Read the model definition and answer for the solid it produces. Units are mm, in the model's axes. Give positions to 0.01 mm unless a question says otherwise; leave off trailing zeros. Write each loop counter-clockwise with the first axis right and the second up, starting at its lowest first coordinate (ties: lowest second). Pieces come first, ordered by that corner, then holes. Notation, with made-up numbers: (-13.75, 45) -> (6.25, 45) arc R16 cw to (6.25, 59) -> close; hole circle Ø8 at (40, 59). An arc over 180 degrees is marked (long way). Use a Markdown table: item, result.
from build123d import *

# Parameters (mm, degrees)
F1_DEPTH = 5
F2_D     = 3
F3_R     = 2.49999


# Not quite as in the source:
# - a fillet or chamfer is up to 0.001 mm smaller than in the source, because OpenCascade refuses the exact size


with BuildPart() as f1:
    # F0 (on Top) → F1 (new body)
    with BuildSketch(Plane.XY):
        Polygon((43.4433006123, 0), (68.4433006123, 0), (68.4433006123, 5), (8.4433006123, 5), (8.4433006123, 0), (40.9433006123, 0), align=None)
    extrude(amount=F1_DEPTH)

    # F2 (through all)
    with Locations(Plane(origin=(0, 0, 0), x_dir=(1, 0, 0), z_dir=(0, 0, -1))):
        with Locations((40.9433006123, -2.5), (65.9433006123, -2.5), (10.9449457377, -2.5)):
            Hole(F2_D / 2)

    # F3 (radius 2.5 in the source; OpenCascade refuses exactly that, so slightly less here)
    f3_edges = [f1.edges().sort_by_distance(p)[0] for p in [
        (8.443301, 0, 2.5),
        (8.443301, 5, 2.5),
        (68.443301, 0, 2.5),
        (68.443301, 5, 2.5),
    ]]
    fillet(f3_edges, radius=F3_R)


solid = f1.part
Item 1: A cutting plane is placed at B-B (y = 1.85). Give the vertices of the cut face in (x, z).
Return value:
| item | result |
|---|---|
| outline | (8.53, 0) -> (9.59, 0) -> (9.59, 5) -> (8.53, 5) -> close; (12.3, 0) -> (39.59, 0) -> (39.59, 5) -> (12.3, 5) -> close; (42.3, 0) -> (64.59, 0) -> (64.59, 5) -> (42.3, 5) -> close; (67.3, 0) -> (68.36, 0) -> (68.36, 5) -> (67.3, 5) -> close |
Item 2: For a pull along X with two mould halves and no side action, classify faces 1 (the face through (38, 3, 5)), 2 (the face through (10.139, 1.235, 2.535)), 3 (the face through (9.2, 4.29, 2.54)) as +X half, -X half, draft (parallel to the pull), parting line (faces both ways), or undercut.
Return value:
| item | result |
|---|---|
| face 1 | draft |
| face 2 | undercut |
| face 3 | -X half |
Item 3: Straight lines are drawn through the part: line 1 along Y through (x, z) = (66, 1.1); line 2 along X through (y, z) = (3.1, 4.55); line 3 along X through (y, z) = (2.05, 3.9). For each, find the intervals that lie inside material, in ascending order. Write a range as [from, to].
Return value:
| item | result |
|---|---|
| line 1 | [0, 1], [4, 5] |
| line 2 | [8.52, 9.57], [12.32, 39.57], [42.32, 64.57], [67.32, 68.37] |
| line 3 | [8.48, 9.51], [12.38, 39.51], [42.37, 64.51], [67.37, 68.4] |
Item 4: A cutting plane is placed at A-A (z = 1.5). Count the separate pieces of the cut face and the enclosed holes in it, then the cut area to 3 significant figures.
Return value:
| item | result |
|---|---|
| separate pieces | 1 |
| enclosed holes | 3 |
| area | 273 mm^2 |
